from build123d import *

# Parameters (mm, degrees)
SKETCH_1_W      = 230
SKETCH_1_H      = 1
EXTRUDE_1_DEPTH = 15
M3X0_5_1_D      = 2.5
M5X0_8_1_D      = 4.2
SKETCH_10_W     = 20
SKETCH_10_H     = 1
EXTRUDE_3_DEPTH = 40
SKETCH_11_W     = 40
SKETCH_11_H     = 1
EXTRUDE_4_DEPTH = 40
M5X0_8_3_D      = 4.2


with BuildPart() as part:
    # ｽｹｯﾁ1 → ﾎﾞｽ - 押し出し1 (new body)
    with BuildSketch(Plane.XY):
        with Locations((115, 0.5)):
            Rectangle(SKETCH_1_W, SKETCH_1_H)
    extrude(amount=EXTRUDE_1_DEPTH)

    # M3x0.5 ねじ穴1 (through all)
    with Locations(Plane(origin=(0, 0, 0), x_dir=(-1, 0, 0), z_dir=(0, -1, 0))):
        with Locations((-9, -8), (-223, -8)):
            Hole(M3X0_5_1_D / 2)

    # M5x0.8 ねじ穴1 (through all)
    with Locations(Plane(origin=(0, 1, 0), x_dir=(1, 0, 0), z_dir=(0, 1, 0))):
        with Locations((30, -8), (200, -8)):
            Hole(M5X0_8_1_D / 2)

    # ｽｹｯﾁ10 → ﾎﾞｽ - 押し出し3 (add)
    with BuildSketch(Plane(origin=(0, 0, 0), x_dir=(-1, 0, 0), z_dir=(0, 0, -1))):
        with Locations((-200, 0.5)):
            Rectangle(SKETCH_10_W, SKETCH_10_H)
    extrude(amount=EXTRUDE_3_DEPTH)

    # ｽｹｯﾁ11 → ﾎﾞｽ - 押し出し4 (add)
    with BuildSketch(Plane(origin=(0, 0, 0), x_dir=(-1, 0, 0), z_dir=(0, 0, -1))):
        with Locations((-20, 0.5)):
            Rectangle(SKETCH_11_W, SKETCH_11_H)
    extrude(amount=EXTRUDE_4_DEPTH)

    # M5x0.8 ねじ穴3 (through all)
    with Locations(Plane(origin=(0, 1, 0), x_dir=(1, 0, 0), z_dir=(0, 1, 0))):
        with Locations((30, 22), (200, 22)):
            Hole(M5X0_8_3_D / 2)


solid = part.part
The model under review builds one solid part; all positions refer to its coordinate system, in mm. Round coordinates to 2 decimals unless told otherwise and drop trailing zeros. Loops run counter-clockwise (first coordinate to the right, second up) from the corner with the lowest first, then second, coordinate; pieces in that order, holes last. Notation, with made-up numbers: (7.25, 48.5) -> (40.25, 48.5) arc R14 cw to (40.25, 55.5) -> close; hole circle Ø7 at (71.5, 79). An arc over 180 degrees is marked (long way). One line per question, with ' | ' between items. Start each with the question number.
Item 1: Add section A-A, the plane z = -22. Write out the cut boundary in (x, y), then the cut area to 3 significant figures.
Item 2: Draft analysis for pull direction X (two halves, no side actions). For faces 1 (the face through (31.548, 0.493, -23.419)), 2 (the face through (91, 1, 6)), state which applies: +X half, -X half, draft (parallel to the pull), parting line (faces both ways), or undercut.
Item 3: Add section B-B, the plane x = 200. Write out the cut boundary in (y, z).
Item 4: For pin 1 (3.5 mm diameter, centred on x = 200, z = -22, fed in from -Y); pin 2 (0.5 mm diameter, centred on x = 83.5, y = 0.5, fed in from -Z); pin 3 (0.5 mm diameter, centred on y = 0.5, z = -12.5, fed in from +X), all flat-tipped, find the tip position at first contact; note any pin that passes through.
Item 5: Add section C-C, the plane y = 0.15. Write out the cut boundary in (x, z).
Item 6: Add section D-D, the plane x = 63. Write out the cut boundary in (y, z), then the cut area to 3 significant figures.
Item 7: Wall thickness on line 1 along X through (y, z) = (0.35, 8); line 2 along Z through (x, y) = (200, 0.2); line 3 along X through (y, z) = (0.45, -22): over which ranges is each line inside the solid? List them lowest first. Write a range as [from, to].
Return value:
1) outline: (0, 0) -> (27.9, 0) -> (27.9, 1) -> (0, 1) -> close; (32.1, 0) -> (40, 0) -> (40, 1) -> (32.1, 1) -> close; (190, 0) -> (197.9, 0) -> (197.9, 1) -> (190, 1) -> close; (202.1, 0) -> (210, 0) -> (210, 1) -> (202.1, 1) -> close | area: 51.6 mm2
2) face 1: undercut | face 2: draft
3) outline: (0, -40) -> (1, -40) -> (1, -24.1) -> (0, -24.1) -> close; (0, -19.9) -> (1, -19.9) -> (1, 5.9) -> (0, 5.9) -> close; (0, 10.1) -> (1, 10.1) -> (1, 15) -> (0, 15) -> close
4) pin 1: passes through | pin 2: stops at z = 0 | pin 3: stops at x = 210
5) outline: (0, -40) -> (40, -40) -> (40, 0) -> (190, 0) -> (190, -40) -> (210, -40) -> (210, 0) -> (230, 0) -> (230, 15) -> (0, 15) -> close; hole circle Ø2.5 at (9, 8); hole circle Ø4.2 at (30, -22); hole circle Ø4.2 at (30, 8); hole circle Ø4.2 at (200, -22); hole circle Ø4.2 at (200, 8); hole circle Ø2.5 at (223, 8)
6) outline: (0, 0) -> (1, 0) -> (1, 15) -> (0, 15) -> close | area: 15.0 mm2
7) line 1: x = [0, 7.75], [10.25, 27.9], [32.1, 197.9], [202.1, 221.75], [224.25, 230] | line 2: z = [-40, -24.1], [-19.9, 5.9], [10.1, 15] | line 3: x = [0, 27.9], [32.1, 40], [190, 197.9], [202.1, 210]
